Autodesk Inventor part; units mm, degrees
ref_plane "YZ Plane" through (0, 0, 0) normal (1, 0, 0) x (0, 1, 0)
ref_plane "XZ Plane" through (0, 0, 0) normal (0, 1, 0) x (-1, 0, 0)
ref_plane "XY Plane" through (0, 0, 0) normal (0, 0, 1) x (1, 0, 0)
sketch "Sketch1" plane through (0, 0, 0) normal (0, 0, 1) x (1, 0, 0)
  line L0 (0, 0) -> (380, 0)
  line L1 (380, 0) -> (380, 54)
  line L2 (380, 54) -> (0, 54)
  line L3 (0, 54) -> (0, 0)
  dimension "d0" = 380
  dimension "d1" = 54
extrude "Extrusion1" add sketch "Sketch1" along normal blind 3
sketch "Sketch2" plane through (0, 0, 3) normal (0, 0, 1) x (1, 0, 0)
  line L0 (0, 54) -> (0, 0)
  line L1 (380, 54) -> (0, 54)
  line L2 (0, 0) -> (380, 0)
  line L3 (380, 0) -> (380, 54)
  point P0 (20, 20)
  point P1 (360, 20)
  dimension "d4" = 20
  dimension "d6" = 20
  dimension "d7" = 20
  dimension "d8" = 20
hole "Hole1" at (20, 20, 3) at (360, 20, 3) direction (0, 0, -1) diameter 7 end through all
sketch "Sketch3" plane through (0, 0, 3) normal (0, 0, 1) x (1, 0, 0)
  line L0 (0, 54) -> (0, 0)
  line L1 (380, 54) -> (0, 54)
  point P0 (153.17, 43.69)
  point P1 (226.83, 43.69)
  dimension "d16" = 73.66
  dimension "d17" = 153.17
  dimension "d18" = 10.31
  dimension "d19" = 10.31
hole "Hole2" at (153.17, 43.69, 3) at (226.83, 43.69, 3) direction (0, 0, -1) diameter 3.5 end through all
properties part number "SupportsheetMonitor" material "Aluminum 6061"
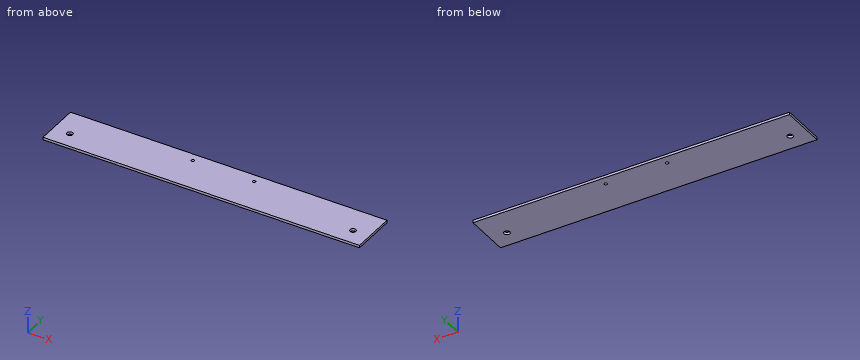
Build history of the part. All positions in model axes, mm. Round coordinates to 2 decimals unless told otherwise and drop trailing zeros. Loops run counter-clockwise (first coordinate to the right, second up) from the corner with the lowest first, then second, coordinate; pieces in that order, holes last.
Item 1: Saw through at A-A (x = 360). List the corners of the cut face in (y, z), then the cut area to 3 significant figures.
Item 2: Drill centre lines: line 1 along X through (y, z) = (20, 2.35); line 2 along Y through (x, z) = (153.17, 0.8); line 3 along Y through (x, z) = (20, 1.2). Where is each one in solid material? Low to high.
Item 3: Pin check, flat tip, straight feed: P1, Ø6.5, axis at x = 20, y = 20, coming from the +Z side. Stop position of the tip, or through.
Item 4: Saw through at B-B (y = 20). List the corners of the cut face in (x, z).
Worked answers:
1. outline: (0, 0) - (16.5, 0) - (16.5, 3) - (0, 3) - close; (23.5, 0) - (54, 0) - (54, 3) - (23.5, 3) - close
1. area: 141 mm2
2. line 1: x = 0 to 16.5, 23.5 to 356.5, 363.5 to 380
2. line 2: y = 0 to 41.94, 45.44 to 54
2. line 3: y = 0 to 16.5, 23.5 to 54
3. P1: passes through
4. outline: (0, 0) - (16.5, 0) - (16.5, 3) - (0, 3) - close; (23.5, 0) - (356.5, 0) - (356.5, 3) - (23.5, 3) - close; (363.5, 0) - (380, 0) - (380, 3) - (363.5, 3) - close
